Check sheet for the modelled part. Datum: model origin and axes. Units: mm. A direction names the side the tool comes from. Round coordinates to 2 decimals unless told otherwise and drop trailing zeros. Loops run counter-clockwise (first coordinate to the right, second up) from the corner with the lowest first, then second, coordinate; pieces in that order, holes last. Notation, with made-up numbers: (46.25, 87) - (94.25, 87) arc R29 ccw to (94.25, 109) - close; hole circle Ø1 at (-18.75, 4). An arc over 180 degrees is marked (long way). Return JSON: item names as keys, results as strings.
from build123d import *

# Parameters (mm, degrees)
SKETCH1_W           = 1.524
SKETCH1_H           = 31.75
BOSS_EXTRUDE1_DEPTH = 2
BOSS_EXTRUDE2_START = 2
SKETCH1_3_W         = 1.524
SKETCH1_3_H         = 31.75
BOSS_EXTRUDE2_DEPTH = 4.7625


with BuildPart() as part:
    # Sketch1 → Boss-Extrude1 (new body)
    with BuildSketch(Plane(origin=(0, 0, 0), x_dir=(1, 0, 0), z_dir=(0, 1, 0))):
        Polygon((3.175, 117.475), (0, 117.475), (0, 111.125), (1.524, 111.125), (1.524, 79.375), (1.524, 47.625), (1.524, 15.875), (1.524, -15.875), (1.524, -47.625), (1.524, -79.375), (1.524, -111.125), (0, -111.125), (0, -117.475), (3.175, -117.475), align=None)
        Polygon((0, 111.125), (0, 117.475), (-3.175, 117.475), (-3.175, -117.475), (0, -117.475), (0, -111.125), (-1.524, -111.125), (-1.524, -79.375), (-1.524, -47.625), (-1.524, -15.875), (-1.524, 15.875), (-1.524, 47.625), (-1.524, 79.375), (-1.524, 111.125), align=None)
        with Locations((-0.762, 95.25)):
            Rectangle(SKETCH1_W, SKETCH1_H)
        with Locations((0.762, 95.25)):
            Rectangle(SKETCH1_W, SKETCH1_H)
        with Locations((0.762, 63.5)):
            Rectangle(SKETCH1_W, SKETCH1_H)
        with Locations((-0.762, 63.5)):
            Rectangle(SKETCH1_W, SKETCH1_H)
        with Locations((-0.762, 31.75)):
            Rectangle(SKETCH1_W, SKETCH1_H)
        with Locations((0.762, 31.75)):
            Rectangle(SKETCH1_W, SKETCH1_H)
        with Locations((0.762, 0)):
            Rectangle(SKETCH1_W, SKETCH1_H)
        with Locations((-0.762, 0)):
            Rectangle(SKETCH1_W, SKETCH1_H)
        with Locations((0.762, -63.5)):
            Rectangle(SKETCH1_W, SKETCH1_H)
        with Locations((-0.762, -63.5)):
            Rectangle(SKETCH1_W, SKETCH1_H)
        with Locations((-0.762, -95.25)):
            Rectangle(SKETCH1_W, SKETCH1_H)
        with Locations((0.762, -95.25)):
            Rectangle(SKETCH1_W, SKETCH1_H)
        with Locations((0.762, -31.75)):
            Rectangle(SKETCH1_W, SKETCH1_H)
        with Locations((-0.762, -31.75)):
            Rectangle(SKETCH1_W, SKETCH1_H)
    extrude(amount=BOSS_EXTRUDE1_DEPTH)

    # Sketch1<3> → Boss-Extrude2 (add)
    with BuildSketch(Plane(origin=(0, 0, 0), x_dir=(1, 0, 0), z_dir=(0, 1, 0)).offset(BOSS_EXTRUDE2_START)):
        with Locations((0.762, 95.25)):
            Rectangle(SKETCH1_3_W, SKETCH1_3_H)
        with Locations((-0.762, 95.25)):
            Rectangle(SKETCH1_3_W, SKETCH1_3_H)
        with Locations((0.762, 31.75)):
            Rectangle(SKETCH1_3_W, SKETCH1_3_H)
        with Locations((-0.762, 31.75)):
            Rectangle(SKETCH1_3_W, SKETCH1_3_H)
        with Locations((0.762, -31.75)):
            Rectangle(SKETCH1_3_W, SKETCH1_3_H)
        with Locations((-0.762, -31.75)):
            Rectangle(SKETCH1_3_W, SKETCH1_3_H)
        with Locations((0.762, -95.25)):
            Rectangle(SKETCH1_3_W, SKETCH1_3_H)
        with Locations((-0.762, -95.25)):
            Rectangle(SKETCH1_3_W, SKETCH1_3_H)
    extrude(amount=BOSS_EXTRUDE2_DEPTH)


solid = part.part
Q1. Sectioned sample at D-D (z = -66). Enter the section's corners in (x, y) (3 decimals), plus the area to 3 significant figures.
Answer key:
{"outline": "(-3.175, 0) - (3.175, 0) - (3.175, 2) - (-3.175, 2) - close", "area": "12.7 mm²"}
Q2. Depth check by flat-ended pin: P1, Ø1.4, axis at y = 4.5, z = -99, coming from the +X side; P2, Ø1.5, axis at x = 0, y = 3.5, coming from the -Z side (3 decimals); P3, Ø3, axis at x = 2, y = 2.5, coming from the -Z side (3 decimals); P4, Ø3.5, axis at x = 0, y = 4.5, coming from the +Z side (3 decimals). Enter the tip coordinate at first touch or a pass-through.
Answer key:
{"P1": "stops at x = 1.52", "P2": "stops at z = -111.125", "P3": "stops at z = -117.475", "P4": "stops at z = 111.125"}
Q3. Scan lines: probe 1 along Z at (x, y) = (-1, 5) (3 decimals); probe 2 along Y at (x, z) = (1.5, -75.5); probe 3 along X at (y, z) = (5, -86). Record each from-to range of solid material in increasing order. Write a range as [from, to].
Answer key:
{"probe 1": "z = [-111.125, -79.375], [-47.625, -15.875], [15.875, 47.625], [79.375, 111.125]", "probe 2": "y = [0, 2]", "probe 3": "x = [-1.52, 1.52]"}
Q4. Tool access check on faces 1 (the face through (0, 0, -2)), 2 (the face through (-1.524, 4, -95)), 3 (the face through (1.524, 4, 32)). Record the directions out of +Z, -Z, +X, -X, +Y, -Y that give a thin tool (end or side, any length) a straight path to the whole face; none if there is none.
Answer key:
{"face 1": "+Z, -Z, +X, -X, -Y", "face 2": "+Z, -Z, -X, +Y", "face 3": "+Z, -Z, +X, +Y"}
Q5. Sectioned sample at C-C (x = 0). Enter the section's corners in (y, z) (1 decimal), plus the area to 3 significant figures.
Answer key:
{"outline": "(0, -117.5) - (2, -117.5) - (2, -111.1) - (6.8, -111.1) - (6.8, -79.4) - (2, -79.4) - (2, -47.6) - (6.8, -47.6) - (6.8, -15.9) - (2, -15.9) - (2, 15.9) - (6.8, 15.9) - (6.8, 47.6) - (2, 47.6) - (2, 79.4) - (6.8, 79.4) - (6.8, 111.1) - (2, 111.1) - (2, 117.5) - (0, 117.5) - close", "area": "1,070 mm²"}
Q6. Sectioned sample at A-A (y = 5.25). Enter the section's corners in (x, z) (3 decimals).
Answer key:
{"outline": "(-1.524, -111.125) - (1.524, -111.125) - (1.524, -79.375) - (-1.524, -79.375) - close; (-1.524, -47.625) - (1.524, -47.625) - (1.524, -15.875) - (-1.524, -15.875) - close; (-1.524, 15.875) - (1.524, 15.875) - (1.524, 47.625) - (-1.524, 47.625) - close; (-1.524, 79.375) - (1.524, 79.375) - (1.524, 111.125) - (-1.524, 111.125) - close"}
Q7. Sectioned sample at B-B (z = 94). Enter the section's corners in (x, y) (1 decimal).
Answer key:
{"outline": "(-3.2, 0) - (3.2, 0) - (3.2, 2) - (1.5, 2) - (1.5, 6.8) - (-1.5, 6.8) - (-1.5, 2) - (-3.2, 2) - close"}
